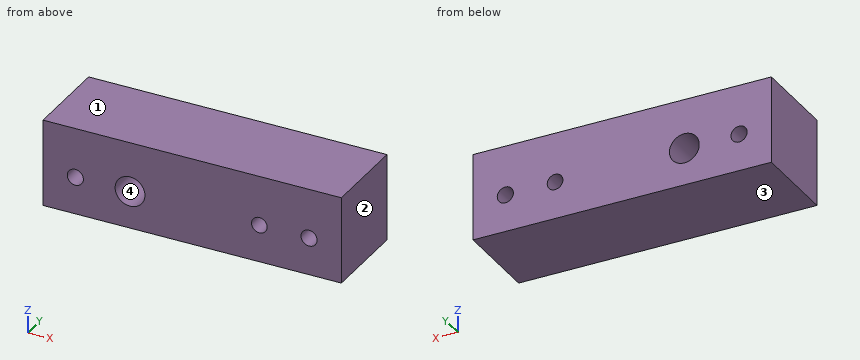
Autodesk Inventor part; units mm, degrees
ref_plane "YZ Plane" through (0, 0, 0) normal (1, 0, 0) x (0, 1, 0)
ref_plane "XZ Plane" through (0, 0, 0) normal (0, 1, 0) x (-1, 0, 0)
ref_plane "XY Plane" through (0, 0, 0) normal (0, 0, 1) x (1, 0, 0)
sketch "스케치1" plane through (0, 0, 0) normal (0, 1, 0) x (-1, 0, 0)
  line L0 (0, 0) -> (12, 0)
  line L1 (12, 0) -> (12, -4)
  line L2 (12, -4) -> (0, -4)
  line L3 (0, -4) -> (0, 0)
  dimension "d0" = 12
  dimension "d1" = 4
extrude "돌출1" add sketch "스케치1" along normal blind 3.5
sketch "스케치2" plane through (0, 3.5, 0) normal (0, 1, 0) x (1, 0, 0)
  line L0 (0, 0) -> (0, 4) construction
  line L1 (0, 2) -> (-12, 2) construction
  line L2 (-12, 4) -> (-12, 0) construction
  point P0 (-1.3, 2)
  point P1 (-3.3, 2)
  point P2 (-8.5, 2)
  point P3 (-10.7, 2)
  dimension "d59" = 1.3
  dimension "d60" = 2.2
  dimension "d61" = 5.2
  dimension "d62" = 1.3
  dimension "d72" = 2
hole "구멍1" at (-10.7, 3.5, -2) at (-1.3, 3.5, -2) direction (0, -1, 0) diameter 0.65 end through all
hole "구멍2" at (-8.5, 3.5, -2) direction (0, -1, 0) diameter 1.2 end through all
hole "구멍3" at (-3.3, 3.5, -2) direction (0, -1, 0) diameter 0.63 end through all
sketch "스케치7" plane through (0, 0, -4) normal (0, 0, -1) x (-1, 0, 0)
  line L0 (12, 0) -> (0, 0)
  line L1 (12, 0) -> (12, 3.5)
  line L2 (0, 3.5) -> (12, 3.5)
  line L3 (0, 0) -> (0, 3.5)
  point P0 (0, 0)
extrude "돌출5" cut sketch "스케치7" against normal blind 0.5
equation "\"G23_F\" = 0.65"
equation "\"G23_M\" = 0.67"
equation "\"Screw_F\" = 1.3"
equation "\"Screw_M\" = 1.6"
properties part number "_3D 인쇄"
Build history of the part. All positions in model axes, mm. Face numbers are marked on the shaded views. Give positions to 0.01 mm unless a question says otherwise; leave off trailing zeros. Loops run counter-clockwise (first coordinate to the right, second up) from the corner with the lowest first, then second, coordinate; pieces in that order, holes last. Notation, with made-up numbers: (29.5, 89) -> (41.5, 89) arc R16 cw to (41.5, 109) -> close; hole circle Ø7 at (-2.5, 61). An arc over 180 degrees is marked (long way). Answer in a Markdown table with one row per item.
Item 1: Probe line 1 along X through (y, z) = (2.05, -2) (3 decimals); line 2 along Z through (x, y) = (-1.3, 1.5) (3 decimals); line 3 along Z through (x, y) = (-8.5, 2.2). List the from-to ranges inside material, lowest first. Write a range as [from, to].
Findings below:
| item | result |
|---|---|
| line 1 | x = [-12, -11.025], [-10.375, -9.1], [-7.9, -3.615], [-2.985, -1.625], [-0.975, 0] |
| line 2 | z = [-3.5, -2.325], [-1.675, 0] |
| line 3 | z = [-3.5, -2.6], [-1.4, 0] |
Item 2: Slice it at A-A on x = -10.7. Write the cut outline in (y, z) (3 decimals).
Findings below:
| item | result |
|---|---|
| outline | (0, -3.5) -> (3.5, -3.5) -> (3.5, -2.325) -> (0, -2.325) -> close; (0, -1.675) -> (3.5, -1.675) -> (3.5, 0) -> (0, 0) -> close |
Item 3: Flat gauge pin, fed straight in: P1, Ø1.1, axis at x = -8.5, z = -2, coming from the +Y side. Where does the tip first touch, or does it go through?
Findings below:
| item | result |
|---|---|
| P1 | passes through |
Item 4: Slice it at D-D on x = -8.5. Write the cut outline in (y, z).
Findings below:
| item | result |
|---|---|
| outline | (0, -3.5) -> (3.5, -3.5) -> (3.5, -2.6) -> (0, -2.6) -> close; (0, -1.4) -> (3.5, -1.4) -> (3.5, 0) -> (0, 0) -> close |
Item 5: Slice it at C-C on z = -1.95. Write the cut outline in (x, y).
Findings below:
| item | result |
|---|---|
| outline | (-12, 0) -> (-11.02, 0) -> (-11.02, 3.5) -> (-12, 3.5) -> close; (-10.38, 0) -> (-9.1, 0) -> (-9.1, 3.5) -> (-10.38, 3.5) -> close; (-7.9, 0) -> (-3.61, 0) -> (-3.61, 3.5) -> (-7.9, 3.5) -> close; (-2.99, 0) -> (-1.62, 0) -> (-1.62, 3.5) -> (-2.99, 3.5) -> close; (-0.98, 0) -> (0, 0) -> (0, 3.5) -> (-0.98, 3.5) -> close |
Item 6: Slice it at B-B on y = 0.3. Write the cut outline in (x, z) (3 decimals).
Findings below:
| item | result |
|---|---|
| outline | (-12, -3.5) -> (0, -3.5) -> (0, 0) -> (-12, 0) -> close; hole circle Ø0.65 at (-10.7, -2); hole circle Ø1.2 at (-8.5, -2); hole circle Ø0.63 at (-3.3, -2); hole circle Ø0.65 at (-1.3, -2) |
Item 7: Mould opens along Z. For the marked faces 1, 2, 3 and 4 say: pulls with the +Z half, pulls with the -Z half, needs draft (parallel to the pull), parting line crosses it, or undercut.
Findings below:
| item | result |
|---|---|
| face 1 | pulls with the +Z half |
| face 2 | needs draft |
| face 3 | pulls with the -Z half |
| face 4 | undercut |
